Model file for the job. Use its own axes, mm. Face numbers are marked on the shaded views. A direction names the side the tool comes from. Round coordinates to 2 decimals unless told otherwise and drop trailing zeros. Loops run counter-clockwise (first coordinate to the right, second up) from the corner with the lowest first, then second, coordinate; pieces in that order, holes last.
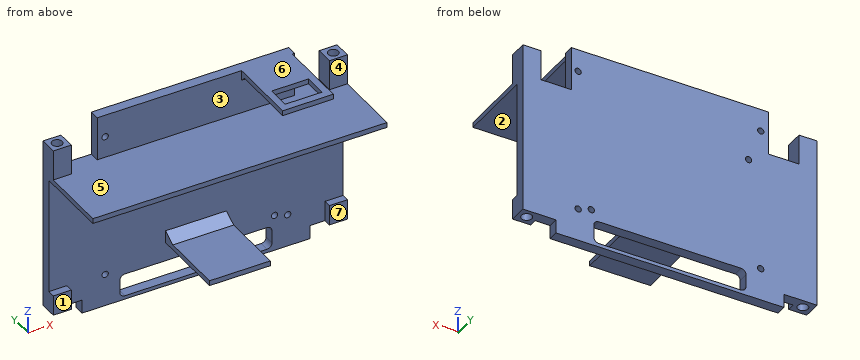
from build123d import *

# Parameters (mm, degrees)
BOSS_EXTRUDE1_DEPTH             = 4
SKETCH3_W                       = 7.1
SKETCH3_H                       = 8
BOSS_EXTRUDE3_DEPTH             = 3
SKETCH4_R                       = 2.05
CUT_EXTRUDE1_DEPTH              = 7
MIRROR2_COPY_1_SKETCH_W         = 7.1
MIRROR2_COPY_1_SKETCH_H         = 8
MIRROR2_COPY_1_DEPTH            = 3
MIRROR2_COPY_2_SKETCH_R         = 2.05
MIRROR2_COPY_2_DEPTH            = 7
SKETCH5_W                       = 60
SKETCH5_H                       = 9
CUT_EXTRUDE2_DEPTH              = 72.37226352
FILLET1_R                       = 2
SKETCH7_W                       = 101.8
SKETCH7_H                       = 1
CUT_EXTRUDE3_DEPTH              = 72.37226352
SKETCH8_W                       = 116
SKETCH8_H                       = 2
BOSS_EXTRUDE4_DEPTH             = 30
SKETCH9_W                       = 12
SKETCH9_H                       = 18
CUT_EXTRUDE4_DEPTH              = 10
SKETCH10_W                      = 7.1
SKETCH10_H                      = 4
BOSS_EXTRUDE5_DEPTH             = 3
SKETCH12_W                      = 1.5
SKETCH12_H                      = 4
BOSS_EXTRUDE6_DEPTH             = 2
SKETCH13_W                      = 36
SKETCH13_H                      = 2
BOSS_EXTRUDE7_DEPTH             = 30
SKETCH14_W                      = 1.5
SKETCH14_H                      = 4
BOSS_EXTRUDE8_DEPTH             = 1
BOSS_EXTRUDE9_REACH             = 79.055
BOSS_EXTRUDE9_DIRECTION_2_REACH = 79.055
SKETCH16_W                      = 20
SKETCH16_H                      = 28
SKETCH16_W_2                    = 14.6
SKETCH16_H_2                    = 9.2
BOSS_EXTRUDE10_DEPTH            = 2.6
SKETCH17_W                      = 12
SKETCH17_H                      = 18
CUT_EXTRUDE5_DEPTH              = 78.054785705
SKETCH18_W                      = 6
SKETCH18_H                      = 6
CUT_EXTRUDE6_DEPTH              = 79.759380394
SKETCH22_R                      = 1.25
CUT_EXTRUDE7_DEPTH              = 4
SKETCH25_W                      = 6
SKETCH25_H                      = 30
CUT_EXTRUDE11_DEPTH             = 10
SKETCH26_W                      = 5.701552738
SKETCH26_H                      = 30.562488548
SKETCH26_W_2                    = 6.53419365
SKETCH26_H_2                    = 28.524331859
CUT_EXTRUDE12_DEPTH             = 78.810282097
CUT_EXTRUDE12_DEPTH_BACK        = 78.810282097
SKETCH27_R                      = 1.25
CUT_EXTRUDE13_DEPTH             = 79.230428862
SKETCH28_W                      = 89.8
SKETCH28_H                      = 0.6
SKETCH28_W_2                    = 77.8
CUT_EXTRUDE14_DEPTH             = 79.230428862
CHAMFER1_SIZE                   = 2


with BuildPart() as part:
    # Sketch1 → Boss-Extrude1 (new body)
    with BuildSketch(Plane(origin=(0, 0, 0), x_dir=(1, 0, 0), z_dir=(0, 1, 0))):
        Polygon((-58, -34), (-50.9, -34), (-50.9, -41), (50.9, -41), (50.9, -34), (58, -34), (58, 34), (50.9, 34), (50.9, 41), (-50.9, 41), (-50.9, 34), (-58, 34), align=None)
    extrude(amount=BOSS_EXTRUDE1_DEPTH)

    # Sketch3 → Boss-Extrude3 (add)
    with BuildSketch(Plane.XZ):
        with Locations((-54.45, -30)):
            Rectangle(SKETCH3_W, SKETCH3_H)
    boss_extrude3 = extrude(amount=BOSS_EXTRUDE3_DEPTH)

    # Sketch4 → Cut-Extrude1 (cut)
    with BuildSketch(Plane(origin=(0, 0, -34), x_dir=(-1, 0, 0), z_dir=(0, 0, -1))):
        with Locations((54.45, 0.5)):
            Circle(SKETCH4_R)
    cut_extrude1 = extrude(amount=-CUT_EXTRUDE1_DEPTH, mode=Mode.SUBTRACT)

    # Mirror1: Boss-Extrude3, Cut-Extrude1 across plane
    add(boss_extrude3.mirror(Plane(origin=(0, 0, 0), x_dir=(0, 0, 1), z_dir=(1, 0, 0))))
    add(cut_extrude1.mirror(Plane(origin=(0, 0, 0), x_dir=(0, 0, 1), z_dir=(1, 0, 0))), mode=Mode.SUBTRACT)

    # Mirror2: Boss-Extrude3, Cut-Extrude1 across plane
    add(boss_extrude3.mirror(Plane.XY))
    add(cut_extrude1.mirror(Plane.XY), mode=Mode.SUBTRACT)

    # Mirror2 copy 1 sketch → Mirror2 copy 1 (add)
    with BuildSketch(Plane(origin=(0, 0, 0), x_dir=(-1, 0, 0), z_dir=(0, -1, 0))):
        with Locations((-54.45, -30)):
            Rectangle(MIRROR2_COPY_1_SKETCH_W, MIRROR2_COPY_1_SKETCH_H)
    extrude(amount=MIRROR2_COPY_1_DEPTH)

    # Mirror2 copy 2 sketch → Mirror2 copy 2 (cut)
    with BuildSketch(Plane.XY.offset(34)):
        with Locations((54.45, 0.5)):
            Circle(MIRROR2_COPY_2_SKETCH_R)
    extrude(amount=-MIRROR2_COPY_2_DEPTH, mode=Mode.SUBTRACT)

    # Sketch5 → Cut-Extrude2 (cut, through all)
    with BuildSketch(Plane(origin=(0, 4, 0), x_dir=(1, 0, 0), z_dir=(0, 1, 0))):
        with Locations((0, 33.5)):
            Rectangle(SKETCH5_W, SKETCH5_H)
    extrude(amount=-CUT_EXTRUDE2_DEPTH, mode=Mode.SUBTRACT)

    # Fillet1
    fillet1_edges = [part.edges().sort_by_distance(p)[0] for p in [
        (-30, 2, -29),
        (-30, 2, -38),
        (30, 2, -38),
        (30, 2, -29),
    ]]
    fillet(fillet1_edges, radius=FILLET1_R)

    # Sketch7 → Cut-Extrude3 (cut, through all)
    with BuildSketch(Plane(origin=(0, 4, 0), x_dir=(1, 0, 0), z_dir=(0, 1, 0))):
        with Locations((0, 40.5)):
            Rectangle(SKETCH7_W, SKETCH7_H)
        with Locations((0, -40.5)):
            Rectangle(SKETCH7_W, SKETCH7_H)
    extrude(amount=-CUT_EXTRUDE3_DEPTH, mode=Mode.SUBTRACT)

    # Sketch8 → Boss-Extrude4 (add)
    with BuildSketch(Plane.XZ):
        with Locations((0, 21)):
            Rectangle(SKETCH8_W, SKETCH8_H)
    extrude(amount=BOSS_EXTRUDE4_DEPTH)

    # Sketch9 → Cut-Extrude4 (cut)
    with BuildSketch(Plane(origin=(0, 4, 0), x_dir=(1, 0, 0), z_dir=(0, 1, 0))):
        with Locations((-44.9, -31)):
            Rectangle(SKETCH9_W, SKETCH9_H)
    extrude(amount=-CUT_EXTRUDE4_DEPTH, mode=Mode.SUBTRACT)

    # Sketch10 → Boss-Extrude5 (add)
    with BuildSketch(Plane.XZ.offset(3)):
        with Locations((-54.45, 24)):
            Rectangle(SKETCH10_W, SKETCH10_H)
        with Locations((54.45, 24)):
            Rectangle(SKETCH10_W, SKETCH10_H)
    extrude(amount=-BOSS_EXTRUDE5_DEPTH)

    # Sketch12 → Boss-Extrude6 (add)
    with BuildSketch(Plane.ZY.offset(51)):
        Polygon((22, -5.8), (22, -16.2), (24.7, -13.5), (24.7, -8.5), align=None)
        with Locations((23.35, -11)):
            Rectangle(SKETCH12_W, SKETCH12_H, mode=Mode.SUBTRACT)
        Polygon((22, -20.8), (22, -31.2), (24.7, -28.5), (24.7, -23.5), align=None)
        with Locations((23.35, -26)):
            Rectangle(SKETCH12_W, SKETCH12_H, mode=Mode.SUBTRACT)
    boss_extrude6 = extrude(amount=-BOSS_EXTRUDE6_DEPTH)

    # Mirror3: Boss-Extrude6 across plane
    add(boss_extrude6.mirror(Plane(origin=(-44.9, 0, 0), x_dir=(0, 0, 1), z_dir=(1, 0, 0))))

    # Sketch13 → Boss-Extrude7 (add)
    with BuildSketch(Plane.XZ):
        with Locations((0, -20.5)):
            Rectangle(SKETCH13_W, SKETCH13_H)
    extrude(amount=BOSS_EXTRUDE7_DEPTH)

    # Sketch14 → Boss-Extrude8 (add, symmetric)
    with BuildSketch(Plane(origin=(0, 0, 0), x_dir=(0, 0, -1), z_dir=(1, 0, 0))):
        Polygon((24.2, -8.5), (21.5, -5.8), (21.5, -16.2), (24.2, -13.5), align=None)
        with Locations((22.85, -11)):
            Rectangle(SKETCH14_W, SKETCH14_H, mode=Mode.SUBTRACT)
    extrude(amount=BOSS_EXTRUDE8_DEPTH, both=True)

    # Boss-Extrude9: up to this face of the body (flat: up to its plane)
    boss_extrude9_end = Plane(part.part.faces().sort_by_distance((-18, -15, -20.5))[0])
    # Sketch15 → Boss-Extrude9 (add, up to the picked face)
    with BuildSketch(Plane(origin=(0, 0, 0), x_dir=(0, 0, -1), z_dir=(1, 0, 0)), mode=Mode.PRIVATE) as boss_extrude9_sk1:
        Polygon((19.5, 0), (19.5, -5), (16.613248654, 0), align=None)
    boss_extrude9_tool1 = split(extrude(boss_extrude9_sk1.sketch, amount=-BOSS_EXTRUDE9_REACH, mode=Mode.PRIVATE), bisect_by=boss_extrude9_end, keep=Keep.BOTH, mode=Mode.PRIVATE)
    add(boss_extrude9_tool1.solids().sort_by(Axis((0, -1.666667, -18.53775), (-1, 0, 0)))[0])

    # Boss-Extrude9 direction 2: up to this face of the body (flat: up to its plane)
    boss_extrude9_direction_2_end = Plane(part.part.faces().sort_by_distance((18, -15, -20.5))[0])
    # Sketch15 → Boss-Extrude9 direction 2 (add, up to the picked face)
    with BuildSketch(Plane(origin=(0, 0, 0), x_dir=(0, 0, -1), z_dir=(1, 0, 0)), mode=Mode.PRIVATE) as boss_extrude9_direction_2_sk1:
        Polygon((19.5, 0), (19.5, -5), (16.613248654, 0), align=None)
    boss_extrude9_direction_2_tool1 = split(extrude(boss_extrude9_direction_2_sk1.sketch, amount=BOSS_EXTRUDE9_DIRECTION_2_REACH, mode=Mode.PRIVATE), bisect_by=boss_extrude9_direction_2_end, keep=Keep.BOTH, mode=Mode.PRIVATE)
    add(boss_extrude9_direction_2_tool1.solids().sort_by(Axis((0, -1.666667, -18.53775), (1, 0, 0)))[0])

    # Sketch16 → Boss-Extrude10 (add)
    with BuildSketch(Plane.XY.offset(40)):
        with Locations((28, -14)):
            Rectangle(SKETCH16_W, SKETCH16_H)
        with Locations((28, -20.4)):
            Rectangle(SKETCH16_W_2, SKETCH16_H_2, mode=Mode.SUBTRACT)
    extrude(amount=-BOSS_EXTRUDE10_DEPTH)

    # Sketch17 → Cut-Extrude5 (cut, through all)
    with BuildSketch(Plane.XZ):
        with Locations((44.9, 31)):
            Rectangle(SKETCH17_W, SKETCH17_H)
    extrude(amount=-CUT_EXTRUDE5_DEPTH, mode=Mode.SUBTRACT)

    # Sketch18 → Cut-Extrude6 (cut, through all)
    with BuildSketch(Plane(origin=(0, 4, 0), x_dir=(1, 0, 0), z_dir=(0, 1, 0))):
        with Locations((47.9, 37)):
            Rectangle(SKETCH18_W, SKETCH18_H)
        with Locations((-47.9, 37)):
            Rectangle(SKETCH18_W, SKETCH18_H)
    extrude(amount=-CUT_EXTRUDE6_DEPTH, mode=Mode.SUBTRACT)

    # Sketch22 → Cut-Extrude7 (cut)
    with BuildSketch(Plane(origin=(0, 4, 0), x_dir=(1, 0, 0), z_dir=(0, 1, 0))):
        with Locations(Location((31, 25, 0), (0, 0, 270))):
            Circle(SKETCH22_R)
        with Locations(Location((-31, -17, 0), (0, 0, 270))):
            Circle(SKETCH22_R)
    extrude(amount=-CUT_EXTRUDE7_DEPTH, mode=Mode.SUBTRACT)

    # Sketch25 → Cut-Extrude11 (cut)
    with BuildSketch(Plane(origin=(0, 0, -21.5), x_dir=(-1, 0, 0), z_dir=(0, 0, -1))):
        with Locations((-15, -15)):
            Rectangle(SKETCH25_W, SKETCH25_H)
        with Locations((15, -15)):
            Rectangle(SKETCH25_W, SKETCH25_H)
    extrude(amount=-CUT_EXTRUDE11_DEPTH, mode=Mode.SUBTRACT)

    # Sketch26 → Cut-Extrude12 (cut, two sides)
    with BuildSketch(Plane.ZY.offset(1)) as cut_extrude12_sk:
        with Locations((-24.350776369, -21.081244274)):
            Rectangle(SKETCH26_W, SKETCH26_H)
        with Locations((25.267096825, -20.06216593)):
            Rectangle(SKETCH26_W_2, SKETCH26_H_2)
    extrude(amount=CUT_EXTRUDE12_DEPTH, mode=Mode.SUBTRACT)
    extrude(cut_extrude12_sk.sketch, amount=-CUT_EXTRUDE12_DEPTH_BACK, mode=Mode.SUBTRACT)

    # Sketch27 → Cut-Extrude13 (cut, through all)
    with BuildSketch(Plane(origin=(0, 4, 0), x_dir=(1, 0, 0), z_dir=(0, 1, 0))):
        with Locations(Location((-35.8, 26.5, 0), (0, 0, 270))):
            Circle(SKETCH27_R)
        with Locations(Location((-35.8, -30.5, 0), (0, 0, 270))):
            Circle(SKETCH27_R)
        with Locations(Location((36.2, -30.5, 0), (0, 0, 270))):
            Circle(SKETCH27_R)
        with Locations(Location((36.2, 26.5, 0), (0, 0, 270))):
            Circle(SKETCH27_R)
    extrude(amount=-CUT_EXTRUDE13_DEPTH, mode=Mode.SUBTRACT)

    # Sketch28 → Cut-Extrude14 (cut, through all)
    with BuildSketch(Plane(origin=(0, 4, 0), x_dir=(1, 0, 0), z_dir=(0, 1, 0))):
        with Locations((0, 39.7)):
            Rectangle(SKETCH28_W, SKETCH28_H)
        with Locations((0, -39.7)):
            Rectangle(SKETCH28_W_2, SKETCH28_H)
    extrude(amount=-CUT_EXTRUDE14_DEPTH, mode=Mode.SUBTRACT)

    # Chamfer1
    chamfer1_edges = [part.edges().sort_by_distance(p)[0] for p in [
        (28, 0, 37.4),
    ]]
    chamfer(chamfer1_edges, length=CHAMFER1_SIZE)


solid = part.part
Q1. Slice it at D-D on x = 54.45. Give the cut face in (y, z).
Q2. Pull direction Z, two halves, no side cores. Call the marked faces 5, 6 and 7: pulls with the +Z half, pulls with the -Z half, needs draft (parallel to the pull), parting line crosses it, or undercut.
Q3. Flat gauge pins, fed straight in: P1, Ø4, axis at x = 24.5, z = 29, coming from the -Y side; P2, Ø4, axis at y = -14.5, z = -18.5, coming from the -X side; P3, Ø8, axis at x = -13, y = -21, coming from the -Z side. Where does each tip first touch, or does it go through?
Q4. Slice it at A-A on z = 17. Give the cut face in (x, y), plus the area to 3 significant figures.
Q5. Slice it at B-B on y = -23.5. Give the cut face in (x, z).
Q6. Probe line 1 (X direction, y = 1.8, z = -26.5); line 2 (Z direction, x = 33, y = -27.5); line 3 (X direction, y = 2.1, z = -25). List the from-to ranges inside material, lowest first.
Q7. Tool access for the marked faces 1, 2, 3 and 4: list every direction of +Z, -Z, +X, -X, +Y, -Y with a clear straight run to the whole face (end or side of a thin tool).
Q8. Slice it at C-C on x = 9. Give the cut face in (y, z), plus the area to 3 significant figures.
Reply:
1. outline: (-30, 20) - (0, 20) - (0, -26) - (-3, -26) - (-3, -34) - (-1.55, -34) - (-1.55, -27) - (2.55, -27) - (2.55, -34) - (4, -34) - (4, 34) - (2.55, 34) - (2.55, 27) - (-1.55, 27) - (-1.55, 34) - (-3, 34) - (-3, 22) - (-30, 22) - close
2. face 5: undercut
2. face 6: pulls with the +Z half
2. face 7: needs draft
3. P1: stops at y = 0
3. P2: stops at x = -12
3. P3: stops at z = -21.5
4. outline: (-58, 0) - (-32.25, 0) - (-32.25, 4) - (-58, 4) - close; (-29.75, 0) - (58, 0) - (58, 4) - (-29.75, 4) - close
4. area: 454 mm2
5. outline: (-58, 20) - (58, 20) - (58, 22) - (-58, 22) - close; (-12, -21.5) - (12, -21.5) - (12, -19.5) - (-12, -19.5) - close; (18, 37.4) - (20.7, 37.4) - (20.7, 39.4) - (18, 39.4) - close; (35.3, 37.4) - (38, 37.4) - (38, 39.4) - (35.3, 39.4) - close
6. line 1: x = -58 to -37.05, -34.55 to 34.95, 37.45 to 58
6. line 2: z = 20 to 22, 37.4 to 39.4
6. line 3: x = -58 to 29.75, 32.25 to 58
7. face 1: -Z, +X, -X, -Y
7. face 2: +X, -X, -Y
7. face 3: -Y
7. face 4: +Z, +X, -X, -Y
8. outline: (-30, -21.5) - (0, -21.5) - (0, -29) - (4, -29) - (4, 39.4) - (0, 39.4) - (0, 22) - (-30, 22) - (-30, 20) - (0, 20) - (0, -16.61) - (-5, -19.5) - (-30, -19.5) - close; (0, -39.4) - (4, -39.4) - (4, -38) - (0, -38) - close
8. area: 406 mm2
